from build123d import *

# Parameters (mm, degrees)
F0_R     = 11.025
F1_DEPTH = 7
F2_R     = 2.5


with BuildPart() as f1:
    # F0 (on Top) → F1 (new body)
    with BuildSketch(Plane.XY):
        with BuildLine():
            ThreePointArc((0, 28), (-17.751289, 10.248711), (-24.248711, -14))
            Line((-24.248711, -14), (0, 28))
        make_face()
        Polygon((-24.248711, -14), (24.248711, -14), (0, 28), align=None)
        Circle(F0_R, mode=Mode.SUBTRACT)
        with BuildLine():
            Line((0, 28), (24.248711, -14))
            ThreePointArc((24.248711, -14), (17.751289, 10.248711), (0, 28))
        make_face()
        with BuildLine():
            ThreePointArc((-24.248711, -14), (0, -20.497423), (24.248711, -14))
            Line((24.248711, -14), (-24.248711, -14))
        make_face()
    extrude(amount=F1_DEPTH)

    # F2
    f2_edges = [f1.edges().sort_by_distance(p)[0] for p in [
        (0, -20.497423, 7),
        (17.751289, 10.248711, 7),
        (-17.751289, 10.248711, 7),
        (0, -20.497423, 0),
        (17.751289, 10.248711, 0),
        (-17.751289, 10.248711, 0),
    ]]
    fillet(f2_edges, radius=F2_R)


solid = f1.part
CAD build for the part. Positions are in the model's coordinates, mm. Give positions to 0.01 mm unless a question says otherwise; leave off trailing zeros. Return JSON: item names as keys, results as strings.
Item 1: Two-plate mould, pull along X, no slides. Class faces 1 (the cylindrical face through (-2.39, -10.763, 3.451)), 2 (the flat face through (-10, -6, 7)), 3 (the cylindrical face through (17.93, 9.94, 3.49)): +X half, -X half, draft (parallel to the pull), parting line (faces both ways), or undercut.
Answer below:
{"face 1": "undercut", "face 2": "draft", "face 3": "+X half"}
Item 2: Drop flat-ended pins along their axis: pin 1 (5 mm diameter, centred on x = -18, y = 12, fed in from +Z); pin 2 (1.5 mm diameter, centred on x = -12, z = 2.5, fed in from +Y); pin 3 (1.5 mm diameter, centred on x = -8.5, y = 19.5, fed in from +Z). Give the stop position or say it passes through.
Answer below:
{"pin 1": "stops at z = 6.74", "pin 2": "stops at y = 19.04", "pin 3": "stops at z = 7"}
Item 3: Drill centre lines: probe 1 along Y at (x, z) = (-8, 2.25); probe 2 along Y at (x, z) = (-8.5, 2.5); probe 3 along X at (y, z) = (5, 5.75). Where is each one in solid material? Low to high.
Answer below:
{"probe 1": "y = -19.82 to -7.59, 7.59 to 22.21", "probe 2": "y = -19.75 to -7.02, 7.02 to 21.77", "probe 3": "x = -20.01 to -9.83, 9.83 to 20.01"}
